Verification items for the finished model (mm, model axes). A direction names the side the tool comes from. Give positions to 0.01 mm unless a question says otherwise; leave off trailing zeros. Loops run counter-clockwise (first coordinate to the right, second up) from the corner with the lowest first, then second, coordinate; pieces in that order, holes last. Notation, with made-up numbers: M 89,86.25 L 117,86.25 A27 ccw 117,115.25 Z; hole C -4,87 d7. An arc over 180 degrees is marked long. Use a Markdown table: item, result.
from build123d import *

# Parameters (mm, degrees)
BOSS_EXTRUDE1_DEPTH = 6
BOSS_EXTRUDE2_DEPTH = 24.6
BOSS_EXTRUDE3_DEPTH = 6


with BuildPart() as part:
    # Sketch1 → Boss-Extrude1 (new body)
    with BuildSketch(Plane.XY):
        with BuildLine():
            Line((0, 0), (20, 0))
            Line((20, 0), (20, 4))
            Line((20, 4), (23.1, 4))
            Line((23.1, 4), (23.1, 11))
            Line((23.1, 11), (18, 11))
            ThreePointArc((18, 11), (10, 19), (2, 11))
            Line((2, 11), (-1.5, 11))
            Line((-1.5, 11), (-1.5, 4))
            Line((-1.5, 4), (0, 4))
            Line((0, 4), (0, 0))
        make_face()
        Polygon((13, 11), (11.5, 13.598076211), (8.5, 13.598076211), (7, 11), (8.5, 8.401923789), (11.5, 8.401923789), align=None, mode=Mode.SUBTRACT)
    extrude(amount=BOSS_EXTRUDE1_DEPTH)

    # Sketch2 → Boss-Extrude2 (add)
    with BuildSketch(Plane.ZY.offset(1.5)):
        with BuildLine():
            Line((6, 4), (6, 5))
            ThreePointArc((6, 5), (6.292893219, 4.292893219), (7, 4))
            Line((7, 4), (6, 4))
        make_face()
        with BuildLine():
            Line((0, 4), (-1, 4))
            ThreePointArc((-1, 4), (-0.292893219, 4.292893219), (0, 5))
            Line((0, 5), (0, 4))
        make_face()
    extrude(amount=-BOSS_EXTRUDE2_DEPTH)

    # Sketch4 → Boss-Extrude3 (add)
    with BuildSketch(Plane.XY.offset(6)):
        with BuildLine():
            Line((23.1, 4), (23.1, 5))
            ThreePointArc((23.1, 5), (23.392893219, 4.292893219), (24.1, 4))
            Line((24.1, 4), (23.1, 4))
        make_face()
        with BuildLine():
            Line((-1.5, 4), (-2.5, 4))
            ThreePointArc((-2.5, 4), (-1.792893219, 4.292893219), (-1.5, 5))
            Line((-1.5, 5), (-1.5, 4))
        make_face()
    extrude(amount=-BOSS_EXTRUDE3_DEPTH)


solid = part.part
(1) Cross-section at B-B on z = 2.75. Record the cut outline in (x, y).
Results below:
| item | result |
|---|---|
| outline | M -2.5,4 L 0,4 L 0,0 L 20,0 L 20,4 L 24.1,4 A1 cw 23.1,5 L 23.1,11 L 18,11 A8 ccw 2,11 L -1.5,11 L -1.5,5 A1 cw Z; hole M 7,11 L 8.5,8.4 L 11.5,8.4 L 13,11 L 11.5,13.6 L 8.5,13.6 Z |
(2) Set-up check for faces 4 (the flat face through (10, 8.402, 3)), 5 (the flat face through (20, 2, 3)), 6 (the flat face through (-1.5, 8, 3)), 7 (the cylindrical face through (10.628, 4.301, 6.285)): record each of +Z, -Z, +X, -X, +Y, -Y from which the full face is reachable in a straight line by a thin tool's end or side.
Results below:
| item | result |
|---|---|
| face 4 | +Z, -Z |
| face 5 | +Z, -Z, +X, -Y |
| face 6 | +Z, -Z, -X, +Y |
| face 7 | +Z, +X, -X, +Y |
(3) Cross-section at A-A on x = 10. Record the cut outline in (y, z), then the cut area to 3 significant figures.
Results below:
| item | result |
|---|---|
| outline | M 0,0 L 4,0 L 4,-1 A1 cw 5,0 L 8.4,0 L 8.4,6 L 5,6 A1 cw 4,7 L 4,6 L 0,6 Z; M 13.6,0 L 19,0 L 19,6 L 13.6,6 Z |
| area | 83.3 mm^2 |
(4) Cross-section at D-D on y = 7.25. Record the cut outline in (x, z).
Results below:
| item | result |
|---|---|
| outline | M -1.5,0 L 23.1,0 L 23.1,6 L -1.5,6 Z |
(5) Material ranges on line 1 (X direction, y = 5.75, z = 2.75); line 2 (X direction, y = 3, z = 2.75); line 3 (Z direction, x = 6.25, y = 12.5), recorded low to high.
Results below:
| item | result |
|---|---|
| line 1 | -1.5 to 23.1 |
| line 2 | 0 to 20 |
| line 3 | 0 to 6 |
(6) Cross-section at C-C on x = 15.25. Record the cut outline in (y, z), then the cut area to 3 significant figures.
Results below:
| item | result |
|---|---|
| outline | M 0,0 L 4,0 L 4,-1 A1 cw 5,0 L 17.04,0 L 17.04,6 L 5,6 A1 cw 4,7 L 4,6 L 0,6 Z |
| area | 103 mm^2 |
(7) Gauge pin test, flat ends, axial feed: P1, Ø2.5, axis at x = 21, z = 2.5, coming from the +Y side; P2, Ø3, axis at x = 9, y = 1.5, coming from the +Z side; P3, Ø7, axis at x = 6, y = 10, coming from the -Z side. Record the tip position at first contact, or that the pin passes through.
Results below:
| item | result |
|---|---|
| P1 | y = 11 |
| P2 | z = 6 |
| P3 | z = 0 |
(8) Draft check along X on faces 1 (the flat face through (0, 2, 3)), 2 (the cylindrical face through (23.385, 4.301, 3.042)), 3 (the flat face through (12.26, 12.28, 2.96)). Enter one of: +X half, -X half, draft (parallel to the pull), parting line (faces both ways), or undercut.
Results below:
| item | result |
|---|---|
| face 1 | -X half |
| face 2 | +X half |
| face 3 | undercut |
